from build123d import *

# Parameters (mm, degrees)
SKETCH1_W           = 75
SKETCH1_H           = 3
BOSS_EXTRUDE1_DEPTH = 200
SKETCH2_R           = 4.9
BOSS_EXTRUDE2_DEPTH = 10
SKETCH3_W           = 5
SKETCH3_H           = 30
CUT_EXTRUDE1_DEPTH  = 1


with BuildPart() as part:
    # Sketch1 → Boss-Extrude1 (new body)
    with BuildSketch(Plane.XY):
        with Locations((37.5, 1.5)):
            Rectangle(SKETCH1_W, SKETCH1_H)
    extrude(amount=BOSS_EXTRUDE1_DEPTH)

    # Sketch2 → Boss-Extrude2 (add)
    with BuildSketch(Plane(origin=(0, 3, 0), x_dir=(1, 0, 0), z_dir=(0, 1, 0))):
        with Locations(Location((12.5, -10, 0), (0, 0, 90))):
            Circle(SKETCH2_R)
        with Locations(Location((52.5, -190, 0), (0, 0, 90))):
            Circle(SKETCH2_R)
    extrude(amount=BOSS_EXTRUDE2_DEPTH)

    # Sketch3 → Cut-Extrude1 (cut)
    with BuildSketch(Plane.XZ):
        with Locations((27.5, 165)):
            Rectangle(SKETCH3_W, SKETCH3_H)
        with Locations((27.5, 115)):
            Rectangle(SKETCH3_W, SKETCH3_H)
        with Locations((27.5, 65)):
            Rectangle(SKETCH3_W, SKETCH3_H)
        with Locations((27.5, 15)):
            Rectangle(SKETCH3_W, SKETCH3_H)
    extrude(amount=-CUT_EXTRUDE1_DEPTH, mode=Mode.SUBTRACT)


solid = part.part
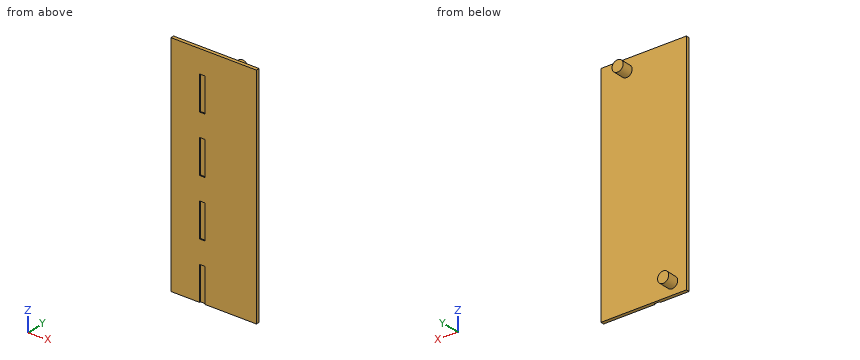
Source: CAD feature listing. Evaluate the final solid. Frame: model axes, mm. Give positions to 0.01 mm unless a question says otherwise; leave off trailing zeros. Write each loop counter-clockwise with the first axis right and the second up, starting at its lowest first coordinate (ties: lowest second). Pieces come first, ordered by that corner, then holes. Notation, with made-up numbers: (32, 21) -> (72, 21) arc R25 ccw to (72, 42) -> close; hole circle Ø8 at (16.5, -29). An arc over 180 degrees is marked (long way). Return JSON: item names as keys, results as strings. Group by question number.
1. Material intervals for line 1 (Z direction, x = 28, y = 0.75); line 2 (Y direction, x = 45.5, z = 31.5); line 3 (Z direction, x = 13, y = 6.75), sorted ascending. Write a range as from..to.
2. Pin query (flat end, axial travel): pin 1 Ø0.5 at (x, y) = (26.5, 0.5) entering from -Z; pin 2 Ø5.5 at (x, z) = (28.5, 162) entering from -Y; pin 3 Ø3 at (x, y) = (56, 8.5) entering from -Z; pin 4 Ø1 at (x, y) = (10, 4) entering from -Z. Return the tip coordinate at first contact, or that it passes through.
3. Section C-C, the plane x = 52.5. Output: boundary loops of the cut face in (y, z).
4. Section A-A, the plane z = 10. Output: boundary loops of the cut face in (x, y), then the cut area to 3 significant figures.
5. Section B-B, the plane y = 6.25. Output: boundary loops of the cut face in (x, z), then the cut area to 3 significant figures.
6. Section D-D, the plane z = 69.5. Output: boundary loops of the cut face in (x, y).
Determined:
{
 "1": {"line 1": "z = 30..50, 80..100, 130..150, 180..200", "line 2": "y = 0..3", "line 3": "z = 5.13..14.87"},
 "2": {"pin 1": "stops at z = 30", "pin 2": "stops at y = 0", "pin 3": "stops at z = 185.53", "pin 4": "stops at z = 5.53"},
 "3": {"outline": "(0, 0) -> (3, 0) -> (3, 185.1) -> (13, 185.1) -> (13, 194.9) -> (3, 194.9) -> (3, 200) -> (0, 200) -> close"},
 "4": {"outline": "(0, 0) -> (25, 0) -> (25, 1) -> (30, 1) -> (30, 0) -> (75, 0) -> (75, 3) -> (17.4, 3) -> (17.4, 13) -> (7.6, 13) -> (7.6, 3) -> (0, 3) -> close", "area": "318 mm2"},
 "5": {"outline": "circle Ø9.8 at (12.5, 10); circle Ø9.8 at (52.5, 190)", "area": "151 mm2"},
 "6": {"outline": "(0, 0) -> (25, 0) -> (25, 1) -> (30, 1) -> (30, 0) -> (75, 0) -> (75, 3) -> (0, 3) -> close"}
}
